```python
from build123d import *

# Parameters (mm, degrees)
F0_W     = 2000
F0_H     = 900
F1_DEPTH = 50
F3_W     = 15
F3_H     = 10
F4_DEPTH = 2000
F5_W     = 15
F5_H     = 10
F6_DEPTH = 2000
F7_W     = 300
F7_H     = 50
F8_DEPTH = 50


with BuildPart() as f1:
    # F0 (on Top) → F1 (new body)
    with BuildSketch(Plane.XY):
        Rectangle(F0_W, F0_H)
    extrude(amount=F1_DEPTH)

    # F3 (on face) → F4 (cut)
    with BuildSketch(Plane.YZ.offset(1000)):
        with Locations((-92.5, 45)):
            Rectangle(F3_W, F3_H)
    extrude(amount=-F4_DEPTH, mode=Mode.SUBTRACT)

    # F5 (on face) → F6 (cut)
    with BuildSketch(Plane.YZ.offset(1000)):
        with Locations((-392.5, 45)):
            Rectangle(F5_W, F5_H)
    extrude(amount=-F6_DEPTH, mode=Mode.SUBTRACT)

    # F7 (on face) → F8 (cut)
    with BuildSketch(Plane.XY.offset(50)):
        with Locations((400, -10)):
            Rectangle(F7_W, F7_H)
    extrude(amount=-F8_DEPTH, mode=Mode.SUBTRACT)


solid = f1.part
```
Read the model definition and answer for the solid it produces. Units are mm, in the model's axes. A direction names the side the tool comes from. Give positions to 0.01 mm unless a question says otherwise; leave off trailing zeros. Order: outer loops, then holes, each group sorted by start corner. A loop starts at its lowest first (then second) coordinate and runs counter-clockwise, first axis right, second up.
(1) For faces 1 (the flat face through (550, -10, 25)), 2 (the flat face through (-14, -450, 25)), determine the directions among +Z, -Z, +X, -X, +Y, -Y from which every point of the face is accessible in a straight line to the end or side of a thin tool.
(2) For a pull along X with two mould halves and no side action, classify faces 3 (the flat face through (-14, -425, 50)), 4 (the flat face through (-1000, -6, 25)), 5 (the flat face through (1000, -6, 25)), 6 (the flat face through (398, -35, 25)) as released by +X, released by -X, zero draft, split by the parting line, or undercut.
(3) Given pin 1 (12 mm diameter, centred on x = 203, y = -92, fed in from +Z), flat-ended and moving along its own axis, determine where the tip first touches the part or whether it passes through.
(4) Find section A-A (x = 300.5). Give the vertices of the cut face in (y, z).
(5) Straight lines are drawn through the part: L1, parallel to Y at x = -159, z = 44; L2, parallel to Y at x = 527.5, z = 41; L3, parallel to X at y = -15, z = 42. For each, find the intervals that lie inside material, in ascending order.
Result sheet:
1. face 1: +Z, -Z
1. face 2: +Z, -Z, +X, -X, -Y
2. face 3: zero draft
2. face 4: released by -X
2. face 5: released by +X
2. face 6: undercut
3. pin 1: stops at z = 40
4. outline: (-450, 0) - (-35, 0) - (-35, 50) - (-85, 50) - (-85, 40) - (-100, 40) - (-100, 50) - (-385, 50) - (-385, 40) - (-400, 40) - (-400, 50) - (-450, 50) - close; (15, 0) - (450, 0) - (450, 50) - (15, 50) - close
5. L1: y = -450 to -400, -385 to -100, -85 to 450
5. L2: y = -450 to -400, -385 to -100, -85 to -35, 15 to 450
5. L3: x = -1000 to 250, 550 to 1000
